Autodesk Inventor part; units mm, degrees
ref_plane "YZ Plane" through (0, 0, 0) normal (1, 0, 0) x (0, 1, 0)
ref_plane "XZ Plane" through (0, 0, 0) normal (0, 1, 0) x (-1, 0, 0)
ref_plane "XY Plane" through (0, 0, 0) normal (0, 0, 1) x (1, 0, 0)
sketch "スケッチ4" plane through (0, 0, 0) normal (0, 0, 1) x (1, 0, 0)
  line L0 (-27, -35) -> (27, -35)
  line L1 (30, -32) -> (30, 32)
  line L2 (27, 35) -> (-27, 35)
  line L3 (-30, 32) -> (-30, -32)
  line L4 (-30, -35) -> (30, 35) construction
  line L5 (30, -35) -> (-30, 35) construction
  line L6 (-25, -30) -> (25, -30) construction
  line L7 (25, -30) -> (25, 30) construction
  line L8 (25, 30) -> (-25, 30) construction
  line L9 (-25, 30) -> (-25, -30) construction
  line L10 (-25, -30) -> (25, 30) construction
  line L11 (25, -30) -> (-25, 30) construction
  circle A0 centre (-25, 30) radius 1.3
  circle A1 centre (25, 30) radius 1.3
  circle A2 centre (25, -30) radius 1.3
  circle A3 centre (-25, -30) radius 1.3
  circle A4 centre (-25, 30) radius 2.6
  circle A5 centre (25, 30) radius 2.6
  circle A6 centre (25, -30) radius 2.6
  circle A7 centre (-25, -30) radius 2.6
  arc A8 (27, -35) -> (30, -32) centre (27, -32) ccw
  arc A9 (-30, -32) -> (-27, -35) centre (-27, -32) ccw
  arc A10 (-27, 35) -> (-30, 32) centre (-27, 32) ccw
  arc A11 (30, 32) -> (27, 35) centre (27, 32) ccw
  line L12 (24, 24) -> (-24, 24) construction
  line L13 (-24, 24) -> (-24, -24) construction
  line L14 (-24, -24) -> (24, -24) construction
  line L15 (24, -24) -> (24, 24) construction
  line L16 (24, 24) -> (-24, -24) construction
  line L17 (-24, 24) -> (24, -24) construction
  circle A12 centre (-24, -24) radius 1.1
  circle A13 centre (-24, 24) radius 1.1
  circle A14 centre (24, -24) radius 1.1
  circle A15 centre (24, 24) radius 1.1
  point P0 (0, 0)
  dimension "d18" = 70
  dimension "d19" = 60
  dimension "d20" = 50
  dimension "d21" = 60
  dimension "d22" = 2.6
  dimension "d30" = 5.2
  dimension "d33" = 3
  dimension "d40" = 48
  dimension "d41" = 48
  dimension "d42" = 2.2
extrude "押し出し4" add sketch "スケッチ4" along normal blind 3 contours A9 L3 A10 L2 A11 L1 A8 L0 | A4 | A5 | A6 | A7
sketch "スケッチ8" plane through (0, 0, 3) normal (0, 0, 1) x (1, 0, 0)
  line L0 (15, 0) -> (-30, 0)
  line L1 (-30, 0) -> (-30, 15.8)
  line L2 (-30, 15.8) -> (15, 15.8)
  line L3 (15, 15.8) -> (15, 0)
  line L4 (-42, 0) -> (42, 0)
  line L5 (-30, 32) -> (-30, -32)
  line L6 (-30, 32) -> (-30, -32)
  line L7 (-30, -4) -> (17, -4)
  line L8 (17, -4) -> (17, 19.8)
  line L9 (17, 19.8) -> (-30, 19.8)
  line L10 (-15, 15.8) -> (-15, 0)
  circle A0 centre (0, 23.9) radius 2
  circle A1 centre (0, -8.1) radius 2
  line L11 (0, -49) -> (0, 49)
  line L12 (15, 7.9) -> (-15, 7.9) construction
  circle A2 centre (-13, -30) radius 0.8
  circle A3 centre (13, -30) radius 0.8
  line L13 (-27, -35) -> (27, -35)
  point P0 (0, 0)
  point P1 (-30, 19.8)
  point P2 (-30, -4)
  dimension "d48" = 15.8
  dimension "d49" = 45
  dimension "d50" = 2
  dimension "d51" = 4
  dimension "d52" = 4
  dimension "d55" = 15
  dimension "d58" = 4
  dimension "d59" = 16
  dimension "d61" = 26
  dimension "d62" = 1.6
  dimension "d63" = 5
extrude "押し出し9" add sketch "スケッチ8" along normal blind 3 contours L0 L11 L7 L5 | L0 L4 L8 L7 L11 | L2 L5 L9 L11 | L3 L2 L11 L9 L8 L4
extrude "押し出し10" cut sketch "スケッチ8" against normal up to surface (3 mm away) contours L0 L1 L2 L10 | A2 | A3
fillet "フィレット2" radius 2 5 edges at (-30, 15.8, 3) (-30, 0, 3) (-15, 7.9, 3) (17, 19.8, 4.5) (17, -4, 4.5)
sketch "スケッチ10" plane through (0, 0, 6) normal (0, 0, 1) x (1, 0, 0)
  circle A0 centre (-25, 17.8) radius 0.8
  circle A1 centre (10, 17.8) radius 0.8
  line L0 (-25, 17.8) -> (10, 17.8) construction
  line L1 (10, 17.8) -> (10, -2) construction
  line L2 (10, -2) -> (-25, -2) construction
  line L3 (-25, -2) -> (-25, 17.8) construction
  circle A2 centre (-25, -2) radius 0.8
  circle A3 centre (10, -2) radius 0.8
  arc A4 (-28, 0) -> (-30, -2) centre (-28, -2) ccw
  line L4 (-30, -2) -> (-30, -4)
  line L5 (-30, -4) -> (15, -4)
  line L6 (17, -2) -> (17, 17.8)
  line L7 (15, 19.8) -> (-30, 19.8)
  line L8 (-30, 19.8) -> (-30, 17.8)
  arc A5 (-30, 17.8) -> (-28, 15.8) centre (-28, 17.8) ccw
  line L9 (-28, 15.8) -> (15, 15.8)
  line L10 (15, 15.8) -> (15, 0)
  line L11 (15, 0) -> (-28, 0)
  circle A6 centre (-25, 17.8) radius 2 construction
  circle A7 centre (10, -2) radius 2 construction
  arc A8 (15, -4) -> (17, -2) centre (15, -2) ccw
  arc A9 (17, 17.8) -> (15, 19.8) centre (15, 17.8) ccw
  point P0 (0, 0)
  point P1 (-30, 18.8)
  dimension "d64" = 1.6
  dimension "d65" = 5
  dimension "d66" = 5
extrude "押し出し11" cut sketch "スケッチ10" against normal up to surface (6 mm away) contours A0 | A1 | A2 | A3
equation "\"d51\" = d52"
properties part number "ThirdPlate"
Check sheet for the modelled part. Datum: model origin and axes. Units: mm. A direction names the side the tool comes from. Coordinates: 2 decimals unless noted, no trailing zeros. Write each loop counter-clockwise with the first axis right and the second up, starting at its lowest first coordinate (ties: lowest second). Pieces come first, ordered by that corner, then holes.
Item 1: Cross-section at B-B on x = 13. Record the boundary of the cut face in (y, z).
Numbers:
outline: (-35, 0) - (-30.8, 0) - (-30.8, 3) - (-35, 3) - close; (-29.2, 0) - (35, 0) - (35, 3) - (19.8, 3) - (19.8, 6) - (15.8, 6) - (15.8, 3) - (0, 3) - (0, 6) - (-4, 6) - (-4, 3) - (-29.2, 3) - close
Item 2: Depth check by flat-ended pin: pin 1 Ø1 at (x, y) = (-23.5, -23.5) entering from +Z; pin 2 Ø0.9 at (y, z) = (4.5, 4) entering from +X; pin 3 Ø2 at (x, y) = (-25, -2) entering from +Z; pin 4 Ø3.5 at (y, z) = (11, 4.5) entering from -X. Enter the tip coordinate at first touch or a pass-through.
Numbers:
pin 1: stops at z = 3
pin 2: stops at x = 17
pin 3: stops at z = 6
pin 4: stops at x = -13.97
Item 3: Scan lines: probe 1 along Y at (x, z) = (12.5, 4.2); probe 2 along Y at (x, z) = (24, 2.45); probe 3 along X at (y, z) = (17.5, 5.05). Record each from-to range of solid material in increasing order.
Numbers:
probe 1: y = -4 to 0, 15.8 to 19.8
probe 2: y = -35 to -30.83, -29.17 to -25.1, -22.9 to 22.9, 25.1 to 29.17, 30.83 to 35
probe 3: x = -29.98 to -25.74, -24.26 to 9.26, 10.74 to 17
Item 4: Cross-section at D-D on y = 2. Record the boundary of the cut face in (x, z), then the cut area to 3 significant figures.
Numbers:
outline: (-15, 0) - (30, 0) - (30, 3) - (17, 3) - (17, 6) - (15, 6) - (15, 3) - (-13, 3) arc R2 ccw to (-15, 1) - close
area: 140 mm2
Item 5: Cross-section at A-A on y = -24. Record the boundary of the cut face in (x, z).
Numbers:
outline: (-30, 0) - (-25.1, 0) - (-25.1, 3) - (-30, 3) - close; (-22.9, 0) - (22.9, 0) - (22.9, 3) - (-22.9, 3) - close; (25.1, 0) - (30, 0) - (30, 3) - (25.1, 3) - close
Item 6: Access from +Z, -Z, +X, -X, +Y, -Y to the whole of each face (thin tool, end or side, straight path). Record for faces 1 (the face through (16.43, 19.2, 4.52)), 2 (the face through (1, 8, 3)), 3 (the face through (-29.4, 16.37, 2.96)), 4 (the face through (23.13, -23.33, 1.48)), 5 (the face through (-30, 25, 2)).
Numbers:
face 1: +Z, +X, +Y
face 2: +Z, -X
face 3: +Z, -Z, -X
face 4: +Z, -Z
face 5: +Z, -Z, -X, +Y, -Y
Item 7: Cross-section at C-C on z = 4.55. Record the boundary of the cut face in (x, y).
Numbers:
outline: (-30, -4) - (15, -4) arc R2 ccw to (17, -2) - (17, 17.8) arc R2 ccw to (15, 19.8) - (-30, 19.8) - (-30, 17.8) arc R2 ccw to (-28, 15.8) - (15, 15.8) - (15, 0) - (-28, 0) arc R2 ccw to (-30, -2) - close; hole circle Ø1.6 at (-25, -2); hole circle Ø1.6 at (-25, 17.8); hole circle Ø1.6 at (10, -2); hole circle Ø1.6 at (10, 17.8)
Item 8: Mould release check, pull along Y, two halves, no side actions. Record for faces 6 (the face through (-7, 19.8, 4)), 7 (the face through (-24.57, 18.475, 3.042)), 8 (the face through (30, 0, 1)), 9 (the face through (-8, -4, 4)): released by +Y, released by -Y, zero draft, split by the parting line, or undercut.
Numbers:
face 6: released by +Y
face 7: undercut
face 8: zero draft
face 9: released by -Y
